For this review, take the finished solid that the model builds, in its own axes (mm). Face numbers are marked on the shaded views. A direction names the side the tool comes from. Give positions to 0.01 mm unless a question says otherwise; leave off trailing zeros. Write each loop counter-clockwise with the first axis right and the second up, starting at its lowest first coordinate (ties: lowest second). Pieces come first, ordered by that corner, then holes.
Q1. We need section C-C (y = -3.25). Give the number of separate pieces and of enclosed holes in the cut face, then the cut area to 3 significant figures.
Q2. We need section B-B (x = -105.5). Write out the cut boundary in (y, z).
Q3. Insertion check: P1, Ø6, axis at x = -84.5, z = -23, coming from the +Y side. The pin has a flat end and moves straight along its axis. Give the tip position at first contact, or say it passes through.
Q4. We need section A-A (z = 33). Write out the cut boundary in (x, y).
Q5. For line 1 (X direction, y = -7, z = -56); line 2 (X direction, y = -8, z = -44); line 3 (X direction, y = -9.25, z = -7), list the stretches that pass through material, from the lowest coordinate up.
Q6. Mouldability with a two-part tool opening along X and no side actions: class the marked faces 1 and 2 as released by +X, released by -X, zero draft, split by the parting line, or undercut.
Q7. Machinability: for the marked faces 3 and 4, which of the approach directions +Z, -Z, +X, -X, +Y, -Y give a long, thin tool a straight path to every point of the face, cutting with its end or side? Answer none if there is none.
Autodesk Fusion 360 part; units mm, degrees
sketch "Sketch1" plane through (0, 0, 0) normal (0, 1, 0) x (1, 0, 0)
  line L0 (-127.5, -64) -> (127.5, -64)
  line L1 (127.5, -64) -> (127.5, 64)
  line L2 (127.5, 64) -> (-127.5, 64)
  line L3 (-127.5, 64) -> (-127.5, -64)
  line L4 (127.5, 0) -> (0, 0) construction
  line L5 (0, 0) -> (0, -64) construction
  circle A0 centre (0, -56) radius 2
  circle A1 centre (119.5, -56) radius 2
  circle A2 centre (119.5, 56) radius 2
  circle A3 centre (0, 56) radius 2
  line L6 (119.5, -56) -> (119.5, 56) construction
  circle A4 centre (-119.5, -56) radius 2
  circle A5 centre (-119.5, 56) radius 2
  line L7 (115.5, -52) -> (6.5, -52)
  line L8 (6.5, -52) -> (6.5, 52)
  line L9 (6.5, 52) -> (115.5, 52)
  line L10 (115.5, 52) -> (115.5, -52)
  line L11 (-6.5, 52) -> (-115.5, 52)
  line L12 (-115.5, 52) -> (-115.5, -52)
  line L13 (-115.5, -52) -> (-6.5, -52)
  line L14 (-6.5, -52) -> (-6.5, 52)
  line L15 (115.5, -20) -> (121.5, -20)
  line L16 (121.5, -20) -> (121.5, 20)
  line L17 (121.5, 20) -> (115.5, 20)
  line L18 (121.5, 0) -> (127.5, 0) construction
  line L19 (-115.5, -20) -> (-121.5, -20)
  line L20 (-121.5, -20) -> (-121.5, 20)
  line L21 (-121.5, 20) -> (-115.5, 20)
  dimension "d4" = 255
  dimension "d5" = 128
  dimension "d8" = 4
  dimension "d9" = 8
  dimension "d10" = 4
  dimension "d11" = 8
  dimension "d12" = 8
  dimension "d13" = 12
  dimension "d14" = 12
  dimension "d15" = 6.5
  dimension "d16" = 12
  dimension "d21" = 40
  dimension "d23" = 6
extrude "Extrude1" add sketch "Sketch1" against normal blind 13.5 contours L0 L1 L2 L3 | A0 | A1 | A2 | A3 | A4 | A5 | L7 L8 L9 L10 | L10 L15 L16 L17 | L11 L12 L13 L14 | L12 L19 L20 L21
extrude "Extrude2" cut sketch "Sketch1" against normal blind 10 contours L7 L8 L9 L10 | L10 L15 L16 L17 | L11 L12 L13 L14 | L12 L19 L20 L21
extrude "Extrude3" cut sketch "Sketch1" against normal blind 10 contours A0 | A1 | A2 | A3 | A4 | A5
fillet "Fillet1" radius 3 16 edges at (115.5, -5, -52) (6.5, -5, -52) (6.5, -5, 52) (115.5, -5, 52) (115.5, -5, 20) (121.5, -5, 20) (121.5, -5, -20) (115.5, -5, -20) (-6.5, -5, 52) (-6.5, -5, -52) (-115.5, -5, -52) (-115.5, -5, -20) (-121.5, -5, -20) (-121.5, -5, 20) (-115.5, -5, 20) (-115.5, -5, 52)
equation "matrixWidth = 128 mm"
equation "matrixLength = 255 mm"
equation "matrixThickness = 13.5 mm"
equation "d4 = matrixLength"
equation "d5 = matrixWidth"
equation "d8 = mHole"
equation "d9 = HoleDist"
equation "d10 = mHole"
equation "d11 = HoleDist"
equation "d12 = HoleDist"
equation "mHole = 4 mm"
equation "HoleDist = 8 mm"
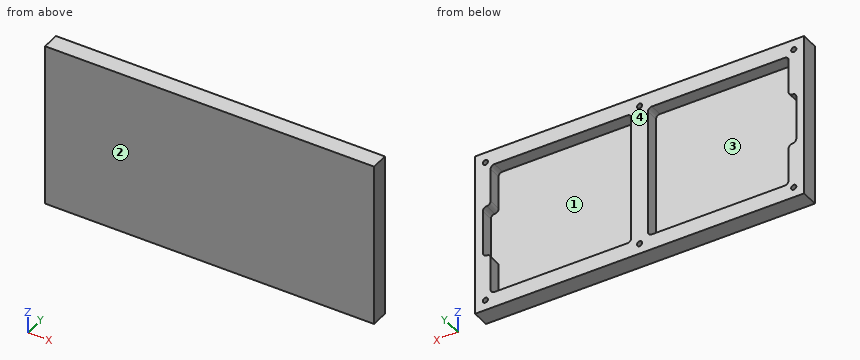
Computed:
1. separate pieces: 1
1. enclosed holes: 8
1. area: 9,430 mm2
2. outline: (-13.5, -64) - (0, -64) - (0, -52) - (-10, -52) - (-10, 52) - (0, 52) - (0, 64) - (-13.5, 64) - close
3. P1: stops at y = -10
4. outline: (-127.5, -13.5) - (127.5, -13.5) - (127.5, 0) - (115.5, 0) - (115.5, -10) - (6.5, -10) - (6.5, 0) - (-6.5, 0) - (-6.5, -10) - (-115.5, -10) - (-115.5, 0) - (-127.5, 0) - close
5. line 1: x = -127.5 to -121.5, -117.5 to -2, 2 to 117.5, 121.5 to 127.5
5. line 2: x = -127.5 to -115.5, -6.5 to 6.5, 115.5 to 127.5
5. line 3: x = -127.5 to -121.5, -6.5 to 6.5, 121.5 to 127.5
6. face 1: undercut
6. face 2: zero draft
7. face 3: +Y
7. face 4: +Z, -Z, +X, -X, +Y
